```python
from build123d import *

# Parameters (mm, degrees)
BOSS_EXTRUDE1_DEPTH = 139.7
SKETCH3_W           = 139.7
SKETCH3_H           = 3.175
BOSS_EXTRUDE2_DEPTH = 3.175
SKETCH4_W           = 3.175
SKETCH4_H           = 9.525
CUT_EXTRUDE1_DEPTH  = 162.644610179
LPATTERN1_COUNT     = 3
LPATTERN1_PITCH     = 55.372
SKETCH5_R           = 1.27
BOSS_EXTRUDE3_DEPTH = 25.4
CUT_EXTRUDE2_DEPTH  = 163.670343529


with BuildPart() as part:
    # Sketch2 → Boss-Extrude1 (new body)
    with BuildSketch(Plane.XY):
        with BuildLine():
            Line((-50.8, 50.8), (-60.325, 50.8))
            Line((-60.325, 50.8), (-60.325, 53.975))
            Line((-60.325, 53.975), (-50.8, 53.975))
            ThreePointArc((-50.8, 53.975), (-12.633911485, 38.166088515), (3.175, 0))
            Line((3.175, 0), (0, 0))
            ThreePointArc((0, 0), (-14.878975516, 35.921024484), (-50.8, 50.8))
        make_face()
    extrude(amount=BOSS_EXTRUDE1_DEPTH)

    # Sketch3 → Boss-Extrude2 (add)
    with BuildSketch(Plane.ZY.offset(60.325)):
        with Locations((69.85, 52.3875)):
            Rectangle(SKETCH3_W, SKETCH3_H)
    extrude(amount=BOSS_EXTRUDE2_DEPTH)

    # Sketch4 → Cut-Extrude1 (cut, through all)
    with BuildSketch(Plane.XZ.offset(-50.8)):
        with Locations((-52.3875, 124.971707481)):
            Rectangle(SKETCH4_W, SKETCH4_H)
    cut_extrude1 = extrude(amount=-CUT_EXTRUDE1_DEPTH, mode=Mode.SUBTRACT)

    # LPattern1: Cut-Extrude1 ×3
    with Locations(*[(0, 0, -i * LPATTERN1_PITCH) for i in range(1, LPATTERN1_COUNT)]):
        add(cut_extrude1, mode=Mode.SUBTRACT)

    # Sketch5 → Boss-Extrude3 (add)
    with BuildSketch(Plane(origin=(0, 53.975, 0), x_dir=(1, 0, 0), z_dir=(0, 1, 0))):
        with Locations(Location((-25.4, -4.7625, 0), (0, 0, 270))):
            Circle(SKETCH5_R)
        with Locations(Location((-26.00240478, -134.669690924, 0), (0, 0, 270))):
            Circle(SKETCH5_R)
    extrude(amount=-BOSS_EXTRUDE3_DEPTH)

    # Sketch6 → Cut-Extrude2 (cut, through all)
    with BuildSketch(Plane.XY.offset(139.7)):
        with BuildLine():
            ThreePointArc((-50.8, 53.975), (-12.633911485, 38.166088515), (3.175, 0))
            ThreePointArc((3.175, 0), (10.303147702, 61.103147702), (-50.8, 53.975))
        make_face()
    extrude(amount=-CUT_EXTRUDE2_DEPTH, mode=Mode.SUBTRACT)


solid = part.part
```
Can you work these out from the model? Positions are in its coordinate system, mm. A direction names the side the tool comes from. Coordinates: 2 decimals unless noted, no trailing zeros. Write each loop counter-clockwise with the first axis right and the second up, starting at its lowest first coordinate (ties: lowest second). Pieces come first, ordered by that corner, then holes. Notation, with made-up numbers: M -10.5,-38.75 L -4.5,-38.75 A11 cw -4.5,-22.75 Z; hole C 83.5,-5.5 d4. An arc over 180 degrees is marked long. Answer as CSV lines item,"result".
Item 1: Imagine slicing it at D-D on x = -44.5. List the corners of the cut face in (y, z) for me, plus the area to 3 significant figures.
Geometry results:
outline,"M 50.41,0 L 53.61,0 L 53.61,139.7 L 50.41,139.7 Z"
area,"447 mm2"
Item 2: On a 3-axis mill with a long thin cutter (end or side, diameter ignored), from which of +Z, -Z, +X, -X, +Y, -Y can I reach the whole of each face in a straight line? I mean faces 1 (the flat face through (-25, 28.575, 5)), 2 (the flat face through (-50.8, 52, 70)), 3 (the flat face through (-57, 53.975, 69)), 4 (the cylindrical face through (-27.24, 36.91, 134.39)). Say none if no direction works.
Geometry results:
face 1,"+Z, -Z, -X, -Y"
face 2,"+Y, -Y"
face 3,"+Z, -Z, +X, -X, +Y"
face 4,"-Y"
Item 3: Imagine slicing it at B-B on y = 41. List the corners of the cut face in (x, z) for me.
Geometry results:
outline,"C -26,134.67 d2.54; C -25.4,4.76 d2.54; M -20.81,0 L -15.7,0 L -15.7,139.7 L -20.81,139.7 Z"
Item 4: We'd pull the mould along X, two halves only. Please class faces 5 (the flat face through (-52, 52, 9.465)), 6 (the flat face through (2, 0, 69)): +X half, -X half, draft (parallel to the pull), parting line (faces both ways), or undercut.
Geometry results:
face 5,"undercut"
face 6,"draft"
Item 5: Please list where these lines run through material, in increasing order: line 1 along Y through (x, z) = (-50.5, 93); line 2 along Y through (x, z) = (-29, 72.5); line 3 along X through (y, z) = (2, 126.5).
Geometry results:
line 1,"y = 50.8 to 53.97"
line 2,"y = 45.88 to 49.38"
line 3,"x = -0.04 to 3.14"
Item 6: Imagine slicing it at C-C on z = 103.5. List the corners of the cut face in (x, y) for me (3 decimals).
Geometry results:
outline,"M -63.5,50.8 L -50.8,50.8 A50.8 cw 0,0 L 3.175,0 A53.975 ccw -50.8,53.975 L -63.5,53.975 Z"
Item 7: Imagine slicing it at A-A on z = 13.5. List the corners of the cut face in (x, y) for me (3 decimals), plus the area to 3 significant figures.
Geometry results:
outline,"M -63.5,50.8 L -53.975,50.8 L -53.975,53.975 L -63.5,53.975 Z; M -50.8,50.8 A50.8 cw 0,0 L 3.175,0 A53.975 ccw -50.8,53.975 Z"
area,"292 mm2"
Item 8: I'm going to push flat-ended pins straight in: P1, Ø5, axis at y = 17, z = 73, coming from the -X side; P2, Ø1, axis at x = -25, z = 95, coming from the -Y side; P3, Ø1, axis at x = -22, z = 111, coming from the +Y side. Where does each tip first touch, or does it pass through?
Geometry results:
P1,"stops at x = -3.89"
P2,"stops at y = 43.46"
P3,"stops at y = 45.96"
